Check sheet for the modelled part. Datum: model origin and axes. Units: mm. Face numbers are marked on the shaded views. Round coordinates to 2 decimals unless told otherwise and drop trailing zeros. Loops run counter-clockwise (first coordinate to the right, second up) from the corner with the lowest first, then second, coordinate; pieces in that order, holes last. Notation, with made-up numbers: (40, 74.5) - (56, 74.5) arc R14 ccw to (56, 99.5) - close; hole circle Ø7 at (17.5, -31.75). An arc over 180 degrees is marked (long way). Put each result on its own line as item: value. Start each with the question number.
Item 1: Draft check along X on the marked faces 1 and 2. Enter one of: pulls with the +X half, pulls with the -X half, needs draft (parallel to the pull), parting line crosses it, or undercut.
Item 2: Section check A-A, the plane z = -124.25. Record the cut outline in (x, y).
Item 3: Material ranges on line 1 along Y through (x, z) = (-60, -118.05); line 2 along Y through (x, z) = (-60, -123.9); line 3 along Y through (x, z) = (95.5, -122.75), recorded low to high.
Item 4: Section check B-B, the plane x = -50. Give the number of separate pieces and of enclosed holes in the cut face, and give its area (3 significant figures).
Item 5: Gauge pin test, flat ends, axial feed: pin 1 Ø2.5 at (x, y) = (-70, 88) entering from +Z (3 decimals); pin 2 Ø1 at (x, y) = (55.5, 49) entering from +Z; pin 3 Ø9.5 at (x, y) = (96, 137) entering from -Z; pin 4 Ø5 at (y, z) = (131, -123.5) entering from +X. Record the tip position at first contact, or that the pin passes through.
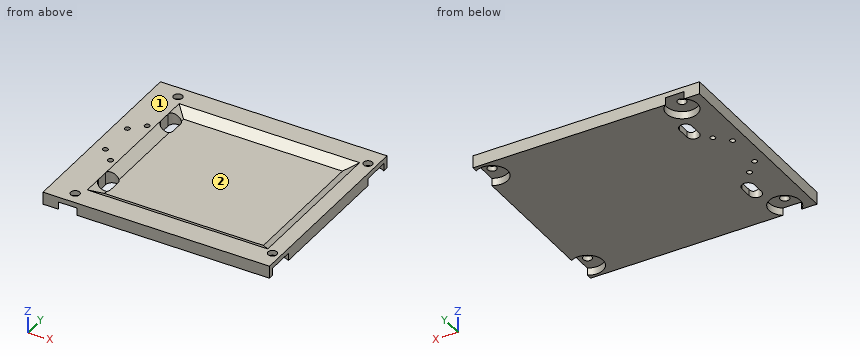
from build123d import *

# Parameters (mm, degrees)
SKETCH014_W         = 182
SKETCH014_H         = 160
PAD007_DEPTH        = 10
HOLE006_D           = 7.1
HOLE006_DEPTH       = 52
HOLE006_CBORE_D     = 25
HOLE006_CBORE_DEPTH = 16
POCKET002_DEPTH     = 29
SKETCH018_W         = 145
SKETCH018_H         = 125
POCKET003_DEPTH     = 5
POCKET003_TAPER     = 60
SKETCH019_R         = 2.1
HOLE007_DEPTH       = 25


with BuildPart() as part:
    # Sketch014 → Pad007 (new body)
    with BuildSketch(Plane.XY):
        with Locations((91, 82)):
            Rectangle(SKETCH014_W, SKETCH014_H)
    extrude(amount=-PAD007_DEPTH)

    # Hole006
    with Locations(Plane(origin=(0, 0, -20), x_dir=(1, 0, 0), z_dir=(0, 0, -1))):
        with Locations((20, -152), (20, -12), (175.5, -147), (175.5, -17)):
            CounterBoreHole(HOLE006_D / 2, HOLE006_CBORE_D / 2, HOLE006_CBORE_DEPTH, depth=HOLE006_DEPTH)

    # Sketch017 → Pocket002 (cut)
    with BuildSketch(Plane.XY):
        with BuildLine():
            ThreePointArc((35, 130), (30, 135), (25, 130))
            Line((25, 130), (25, 120))
            ThreePointArc((25, 120), (30, 115), (35, 120))
            Line((35, 130), (35, 120))
        make_face()
        with BuildLine():
            ThreePointArc((35, 45), (30, 50), (25, 45))
            Line((25, 45), (25, 35))
            ThreePointArc((25, 35), (30, 30), (35, 35))
            Line((35, 45), (35, 35))
        make_face()
    extrude(amount=-POCKET002_DEPTH, mode=Mode.SUBTRACT)

    # Sketch018 → Pocket003 (cut)
    with BuildSketch(Plane.XY):
        with Locations((97.5, 82.5)):
            Rectangle(SKETCH018_W, SKETCH018_H)
    extrude(amount=-POCKET003_DEPTH, taper=POCKET003_TAPER, mode=Mode.SUBTRACT)

    # Sketch019 → Hole007 (cut)
    with BuildSketch(Plane.XY.offset(-20)):
        with Locations((20, 60)):
            Circle(SKETCH019_R)
        with Locations((20, 110)):
            Circle(SKETCH019_R)
        with Locations((10, 100)):
            Circle(SKETCH019_R)
        with Locations((10, 70)):
            Circle(SKETCH019_R)
    extrude(amount=HOLE007_DEPTH, mode=Mode.SUBTRACT)


with BuildPart() as part_1:
    # Body005 placement: moved
    add(part.part.moved(Location((-80, -12, -116))))


solid = part_1.part
Check result:
1. face 1: needs draft
1. face 2: undercut
2. outline: (-80, -10) - (-67.5, -10) arc R12.5 cw (long way) to (-52.5, -10) - (102, -10) - (102, -5.68) arc R12.5 cw (long way) to (102, 15.68) - (102, 124.32) arc R12.5 cw (long way) to (102, 145.68) - (102, 150) - (-52.5, 150) arc R12.5 cw (long way) to (-67.5, 150) - (-80, 150) - close; hole circle Ø4.2 at (-70, 58); hole circle Ø4.2 at (-70, 88); hole circle Ø4.2 at (-60, 48); hole circle Ø4.2 at (-60, 98); hole (-55, 23) arc R5 ccw to (-45, 23) - (-45, 33) arc R5 ccw to (-55, 33) - close; hole (-55, 108) arc R5 ccw to (-45, 108) - (-45, 118) arc R5 ccw to (-55, 118) - close
3. line 1: -10 to -3.55, 3.55 to 45.9, 50.1 to 95.9, 100.1 to 136.45, 143.55 to 150
3. line 2: 12.5 to 45.9, 50.1 to 95.9, 100.1 to 127.5
3. line 3: -10 to -7.5, 17.5 to 122.5, 147.5 to 150
4. separate pieces: 3
4. enclosed holes: 0
4. area: 789 mm²
5. pin 1: through
5. pin 2: z = -121
5. pin 3: z = -120
5. pin 4: x = 84.82
